Check sheet for the drawn part. Datum: minimum x, y, z corner. Units: mm. A direction names the side the tool comes from. Coordinates: 2 decimals unless noted, no trailing zeros. Loops run counter-clockwise (first coordinate to the right, second up) from the corner with the lowest first, then second, coordinate; pieces in that order, holes last. Notation, with made-up numbers: (-1, 86.25) - (25, 86.25) arc R22 cw to (25, 122.25) - close; hole circle Ø11 at (-37.75, 86.25). An arc over 180 degrees is marked (long way). Answer as CSV lines item,"result". Start each with the question number.
1. Cross-section at A-A (y = 8.5). State how many separate pieces and enclosed holes the cut face has.
2. Set-up check for the marked faces 1 and 2: record each of +Z, -Z, +X, -X, +Y, -Y from which the full face is reachable in a straight line by a thin tool's end or side.
3. Material ranges on line 1 (Y direction, x = 4.75, z = 43); line 2 (X direction, y = 18, z = 32) (1 decimal); line 3 (Z direction, x = 8.5, y = 10), recorded low to high. Write a range as [from, to].
4. Cross-section at D-D (z = 14.5). Enter the section's corners in (x, y) (1 decimal).
5. Release check for a two-part mould opening along Z. For the marked faces 3, 4, 5 and 6 record: pulls with the +Z half, pulls with the -Z half, needs draft (parallel to the pull), parting line crosses it, or undercut.
6. Cross-section at B-B (x = 5.75). Enter the section's corners in (y, z).
7. Gauge pin test, flat ends, axial feed: P1, Ø6, axis at x = 7, y = 28, coming from the -Z side; P2, Ø6, axis at x = 12, z = 24.5, coming from the -Y side; P3, Ø8.5, axis at y = 9.22, z = 29.32, coming from the -X side (1 decimal). Record the tip position at first contact, or that the pin passes through.
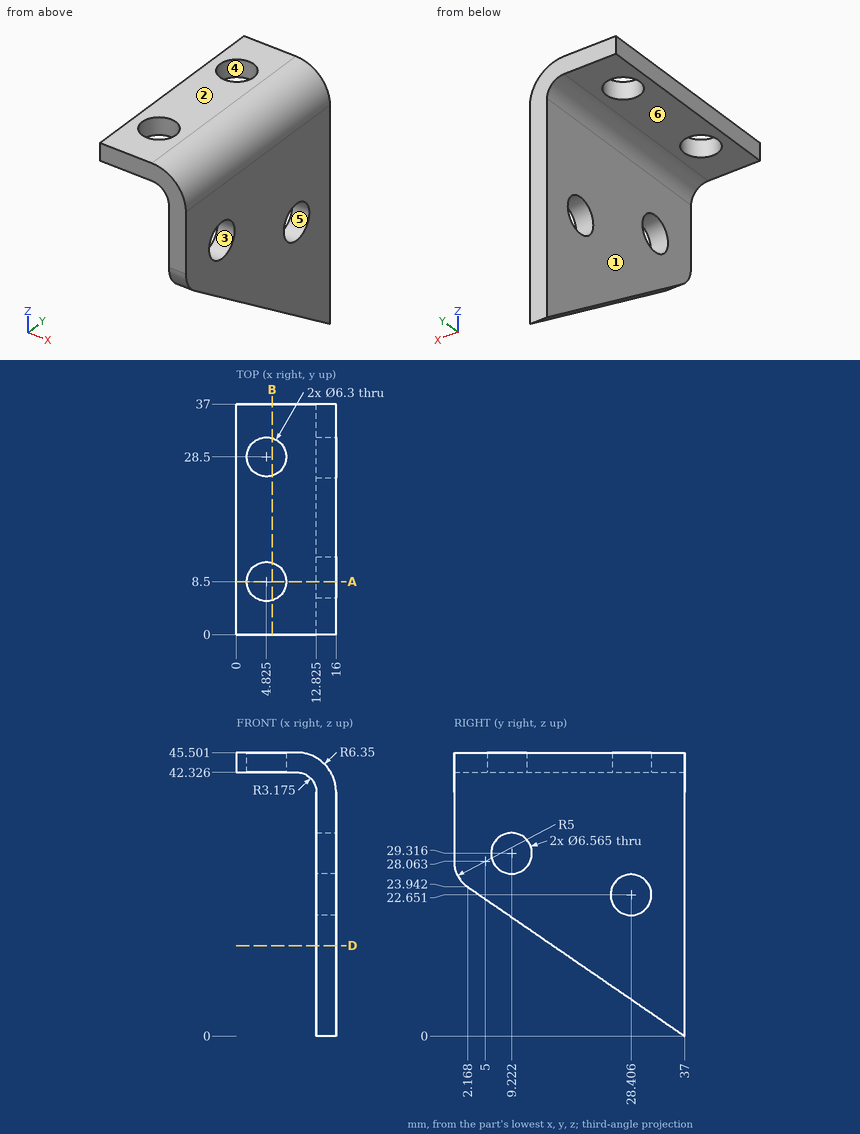
Values follow:
1,separate pieces,"3"
1,enclosed holes,"0"
2,face 1,"-Z, -X, +Y, -Y"
2,face 2,"+Z, +X, -X, +Y, -Y"
3,line 1,"y = [0, 5.35], [11.65, 25.35], [31.65, 37]"
3,line 2,"x = [12.8, 16]"
3,line 3,"z = [42.33, 45.5]"
4,outline,"(12.8, 15.9) - (16, 15.9) - (16, 37) - (12.8, 37) - close"
5,face 3,"undercut"
5,face 4,"needs draft"
5,face 5,"undercut"
5,face 6,"pulls with the -Z half"
6,outline,"(0, 42.33) - (5.49, 42.33) - (5.49, 45.5) - (0, 45.5) - close; (11.51, 42.33) - (25.49, 42.33) - (25.49, 45.5) - (11.51, 45.5) - close; (31.51, 42.33) - (37, 42.33) - (37, 45.5) - (31.51, 45.5) - close"
7,P1,"stops at z = 42.31"
7,P2,"stops at y = 0.05"
7,P3,"stops at x = 12.8"
